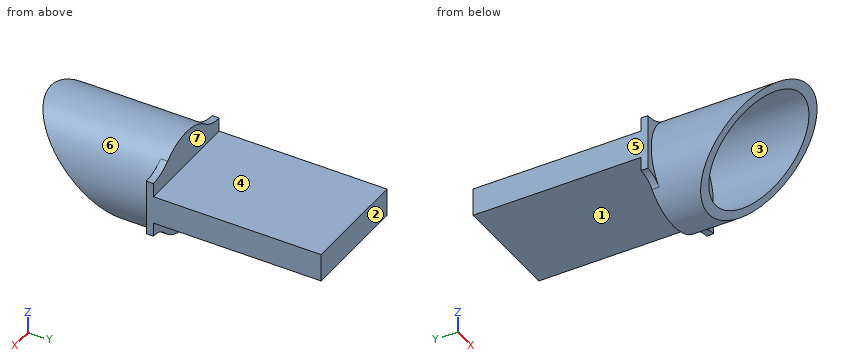
from build123d import *

# Parameters (mm, degrees)
CUT_EXTRUDE1_DEPTH      = 1054.2364613417774
CUT_EXTRUDE1_DEPTH_BACK = 1054.2364613417774
SHELL1_OUTLINE_W        = 19.594743879
SHELL1_OUTLINE_H        = 51.88948775799986
BOSS_EXTRUDE1_DEPTH     = 3.175
SKETCH5_W               = 50.79999999999999
SKETCH5_H               = 12.699999999999998
BOSS_EXTRUDE2_DEPTH     = 76.2


# Read off the part's stored shape, not the designer's step: Shell1
with BuildPart() as part:
    # Sketch2 → Revolve1 (revolve)
    with BuildSketch(Plane(origin=(0, 0, 0), x_dir=(0, 0, -1), z_dir=(1, 0, 0))):
        Polygon((1.0414000000000794, 1052.7210512242139), (-21.7283438789312, 1052.7210512242139), (-21.7283438789312, 994.4815634663521), (1.0414000000000847, 994.4815634663521), align=None)
    revolve(axis=Axis((0, 1052.7210512242139, -1.0414000000000794), (0, -1, -9e-17)))

    # Sketch3 → Cut-Extrude1 (cut, two sides: drawn at the far end of the back side and taken through both)
    with BuildSketch(Plane(origin=(0, 0, 0), x_dir=(0, 0, -1), z_dir=(1, 0, 0)).offset(-CUT_EXTRUDE1_DEPTH_BACK)):
        Polygon((-21.7283438789312, 994.4815634663521), (23.811143878931354, 1040.0210512242138), (23.811143878931365, 994.4815634663521), align=None)
    extrude(amount=CUT_EXTRUDE1_DEPTH + CUT_EXTRUDE1_DEPTH_BACK, mode=Mode.SUBTRACT)

    # Shell1 outline → Shell1 (revolve, cut)
    with BuildSketch(Plane.XY.offset(-1.0414)):
        with Locations((9.7973719395, 1023.601307345)):
            Rectangle(SHELL1_OUTLINE_W, SHELL1_OUTLINE_H)
    revolve(axis=Axis((0, 0, -1.0414), (0, 1, 0)), mode=Mode.SUBTRACT)

    # Sketch4 → Boss-Extrude1 (add)
    with BuildSketch(Plane(origin=(0, 1052.7210512242139, 9.407e-14), x_dir=(1, 0, 0), z_dir=(0, 1, 0))):
        with BuildLine():
            Line((25.4, 12.700000000000092), (25.4, -12.699999999999907))
            ThreePointArc((25.4, -12.699999999999907), (19.547591344304465, -13.709181649641387), (14.371169963720073, -16.62016024211882))
            ThreePointArc((14.371169963720073, -16.62016024211882), (-8.72e-15, -21.72834387893111), (-14.371169963720085, -16.620160242118818))
            ThreePointArc((-14.371169963720085, -16.620160242118818), (-19.54759134430447, -13.709181649641383), (-25.4, -12.699999999999907))
            Line((-25.4, -12.699999999999907), (-25.4, 12.700000000000092))
            ThreePointArc((-25.4, 12.700000000000092), (-20.663631299775105, 13.690635523953107), (-16.72131200571086, 16.496462637200914))
            ThreePointArc((-16.72131200571086, 16.496462637200914), (1.39e-15, 23.811143878931446), (16.72131200571086, 16.496462637200906))
            ThreePointArc((16.72131200571086, 16.496462637200906), (20.663631299775105, 13.690635523953098), (25.4, 12.700000000000092))
        make_face()
    extrude(amount=BOSS_EXTRUDE1_DEPTH)

    # Sketch5 → Boss-Extrude2 (add)
    with BuildSketch(Plane(origin=(0, 1055.8960512242138, 0), x_dir=(1, 0, 0), z_dir=(0, 1, 0))):
        Rectangle(SKETCH5_W, SKETCH5_H)
    extrude(amount=BOSS_EXTRUDE2_DEPTH)


solid = part.part
Verification items for the finished model (mm, model axes). Face numbers are marked on the shaded views. A direction names the side the tool comes from. Give positions to 0.01 mm unless a question says otherwise; leave off trailing zeros. Loops run counter-clockwise (first coordinate to the right, second up) from the corner with the lowest first, then second, coordinate; pieces in that order, holes last. Notation, with made-up numbers: (37, 39.5) - (62, 39.5) arc R31 ccw to (62, 63.5) - close; hole circle Ø2 at (-20.75, -29.5). An arc over 180 degrees is marked (long way). Write each question's results on one line, items separated by ' | '.
1) Sectioned sample at C-C on x = -2. Record the boundary of the cut face in (y, z).
Solution:
outline: (994.57, 21.64) - (997.76, 18.45) - (1049.55, 18.45) - (1049.55, -20.53) - (1036.74, -20.53) - (1039.93, -23.72) - (1055.9, -23.72) - (1055.9, -6.35) - (1132.1, -6.35) - (1132.1, 6.35) - (1055.9, 6.35) - (1055.9, 21.64) - close
2) Depth check by flat-ended pin: P1, Ø12, axis at x = -6, z = 0, coming from the -Y side; P2, Ø15, axis at x = 11.5, y = 1089.5, coming from the -Z side; P3, Ø6, axis at y = 1032, z = 8.5, coming from the -X side. Enter the tip coordinate at first touch or a pass-through.
Solution:
P1: y = 1049.55 | P2: z = -6.35 | P3: x = -21.81
3) Sectioned sample at B-B on y = 1058.5. Record the boundary of the cut face in (x, z), plus the area to 3 significant figures.
Solution:
outline: (-25.4, -6.35) - (25.4, -6.35) - (25.4, 6.35) - (-25.4, 6.35) - close | area: 645 mm2
4) Sectioned sample at A-A on x = -9.5. Record the boundary of the cut face in (y, z), plus the area to 3 significant figures.
Solution:
outline: (996.56, 19.65) - (1000.11, 16.1) - (1049.55, 16.1) - (1049.55, -18.18) - (1034.39, -18.18) - (1037.94, -21.73) - (1055.9, -21.73) - (1055.9, -6.35) - (1132.1, -6.35) - (1132.1, 6.35) - (1055.9, 6.35) - (1055.9, 19.65) - close | area: 1,460 mm2
5) Material ranges on L1, parallel to Y at x = 10.5, z = -9.5; L2, parallel to X at y = 1050.5, z = 0; L3, parallel to Y at x = -8.5, z = 0, recorded low to high. Write a range as from..to.
Solution:
L1: 1049.55..1055.9 | L2: -22.75..22.75 | L3: 1049.55..1132.1
6) Mould release check, pull along Z, two halves, no side actions. Record for the marked faces 1, 2, 3 and 4: pulls with the +Z half, pulls with the -Z half, needs draft (parallel to the pull), parting line crosses it, or undercut.
Solution:
face 1: pulls with the -Z half | face 2: needs draft | face 3: undercut | face 4: pulls with the +Z half
7) Tool access check on the marked faces 5, 6 and 7. Record the directions out of +Z, -Z, +X, -X, +Y, -Y that give a thin tool (end or side, any length) a straight path to the whole face; none if there is none.
Solution:
face 5: +Z, -Z, -X, +Y, -Y | face 6: -Y | face 7: +Z, +X, -X, +Y
